```python
from build123d import *

# Parameters (mm, degrees)
F0_W     = 90.075135231
F0_H     = 62.6202728599
F1_DEPTH = 30.226
F2_R     = 21.4623585695
F3_R     = 5.08
F4_R     = 5.08


with BuildPart() as f1:
    # F0 (on Top) → F1 (new body)
    with BuildSketch(Plane.XY):
        with Locations((-2.6347637177, -21.8688407913)):
            Rectangle(F0_W, F0_H)
    extrude(amount=F1_DEPTH)

    # F2
    f2_edges = [f1.edges().sort_by_distance(p)[0] for p in [
        (-2.634764, -53.178977, 0),
    ]]
    fillet(f2_edges, radius=F2_R)

    # F3
    f3_edges = [f1.edges().sort_by_distance(p)[0] for p in [
        (42.402804, -11.137662, 0),
        (-47.672331, -11.137662, 0),
    ]]
    fillet(f3_edges, radius=F3_R)

    # F4
    f4_edges = [f1.edges().sort_by_distance(p)[0] for p in [
        (-2.634764, -53.178977, 21.462359),
        (-42.592331, -53.178977, 25.844179),
        (37.322804, -53.178977, 25.844179),
        (-2.634764, -53.178977, 30.226),
        (-42.592331, -46.892798, 6.286179),
        (37.322804, -46.892798, 6.286179),
        (-2.634764, -31.716619, 0),
    ]]
    fillet(f4_edges, radius=F4_R)


solid = f1.part
```
Read the model definition and answer for the solid it produces. Units are mm, in the model's axes. Coordinates: 2 decimals unless noted, no trailing zeros. Loops run counter-clockwise (first coordinate to the right, second up) from the corner with the lowest first, then second, coordinate; pieces in that order, holes last. Notation, with made-up numbers: (5.25, 65) - (27.25, 65) arc R19 ccw to (27.25, 82) - close; hole circle Ø2 at (31, 29). An arc over 180 degrees is marked (long way). Answer in a Markdown table with one row per item.
1. Straight lines are drawn through the part: line 1 (X direction, y = -19, z = 5); line 2 (Y direction, x = -35, z = 4); line 3 (Y direction, x = -37, z = 10.5). For each, find the intervals that lie inside material, in ascending order.
Conclusion:
| item | result |
|---|---|
| line 1 | x = -47.67 to 42.4 |
| line 2 | y = -44.19 to 9.44 |
| line 3 | y = -50.17 to 9.44 |
2. Find section A-A, the plane x = 27.5. Write down the section's boundary in (y, z), then the cut area to 3 significant figures.
Conclusion:
| item | result |
|---|---|
| outline | (-53.18, 21.46) arc R21.46 ccw to (-31.72, 0) - (9.44, 0) - (9.44, 30.23) - (-48.1, 30.23) arc R5.08 ccw to (-53.18, 25.15) - close |
| area | 1,790 mm² |
3. Given pin 1 (1 mm diameter, centred on x = -13, z = 6.5, fed in from -Y), flat-ended and moving along its own axis, determine where the tip first touches the part or whether it passes through.
Conclusion:
| item | result |
|---|---|
| pin 1 | stops at y = -47.57 |
